Read the model definition and answer for the solid it produces. Units are mm, in the model's axes. A direction names the side the tool comes from. Round coordinates to 2 decimals unless told otherwise and drop trailing zeros. Loops run counter-clockwise (first coordinate to the right, second up) from the corner with the lowest first, then second, coordinate; pieces in that order, holes last. Notation, with made-up numbers: (39.5, 5) -> (64.5, 5) arc R25 cw to (64.5, 26) -> close; hole circle Ø11 at (-4.75, -11.75). An arc over 180 degrees is marked (long way). Put each result on its own line as item: value.
from build123d import *

# Parameters (mm, degrees)
F0_R     = 6.75
F1_DEPTH = 8
F3_DEPTH = 8.001


with BuildPart() as f1:
    # F0 (on Front) → F1 (new body)
    with BuildSketch(Plane.XZ):
        with Locations((-22.467263, 19.054513)):
            Circle(F0_R)
    extrude(amount=F1_DEPTH)

    # F2 (on face) → F3 (cut, through all)
    with BuildSketch(Plane.XZ.offset(8)):
        with BuildLine():
            Line((-22.467263, 20.554513), (-22.467263, 24.554513))
            ThreePointArc((-22.467263, 24.554513), (-24.660383, 24.098344), (-26.489708, 22.805504))
            Line((-26.489708, 22.805504), (-23.564294, 20.077511))
            ThreePointArc((-23.564294, 20.077511), (-23.065387, 20.430104), (-22.467263, 20.554513))
        make_face()
        with BuildLine():
            Line((-21.040678, 19.518039), (-17.236452, 20.754107))
            ThreePointArc((-17.236452, 20.754107), (-18.348007, 22.698924), (-20.142863, 24.039206))
            Line((-20.142863, 24.039206), (-21.833336, 20.413975))
            ThreePointArc((-21.833336, 20.413975), (-21.343829, 20.048443), (-21.040678, 19.518039))
        make_face()
        with BuildLine():
            ThreePointArc((-19.234444, 14.60492), (-17.728303, 16.263052), (-17.008259, 18.384232))
            Line((-17.008259, 18.384232), (-20.978444, 18.871709))
            ThreePointArc((-20.978444, 18.871709), (-21.174819, 18.293206), (-21.585585, 17.840988))
            Line((-21.585585, 17.840988), (-19.234444, 14.60492))
        make_face()
        with BuildLine():
            ThreePointArc((-25.700082, 14.60492), (-23.657681, 13.684885), (-21.417814, 13.655564))
            Line((-21.417814, 13.655564), (-22.18105, 17.582073))
            ThreePointArc((-22.18105, 17.582073), (-22.791922, 17.590069), (-23.348941, 17.840988))
            Line((-23.348941, 17.840988), (-25.700082, 14.60492))
        make_face()
        with BuildLine():
            Line((-23.893848, 19.518039), (-27.698074, 20.754107))
            ThreePointArc((-27.698074, 20.754107), (-27.941942, 18.527362), (-27.277671, 16.388061))
            Line((-27.277671, 16.388061), (-23.779193, 18.327299))
            ThreePointArc((-23.779193, 18.327299), (-23.960357, 18.910745), (-23.893848, 19.518039))
        make_face()
    extrude(amount=-F3_DEPTH, mode=Mode.SUBTRACT)


solid = f1.part
Item 1: Flat-ended cylindrical pins translate along their axes: pin 1 Ø3 at (y, z) = (-6.5, 14) entering from -X; pin 2 Ø6 at (x, z) = (-22.5, 23) entering from -Y; pin 3 Ø4.5 at (y, z) = (-6, 22.5) entering from -X; pin 4 Ø1 at (x, y) = (-24.5, -4.5) entering from +Z. Find the tip coordinate at first contact, or state that the pin passes through.
Derived:
pin 1: stops at x = -28.21
pin 2: stops at y = -8
pin 3: stops at x = -29.11
pin 4: stops at z = 25.63
Item 2: Which of the six approach directions +Z, -Z, +X, -X, +Y, -Y give full straight-line access (tool end or side, diameter ignored) to faces 3 (the flat face through (-25.553, -4.056, 17.344)), 4 (the flat face through (-23, 0, 19))?
Derived:
face 3: +Y, -Y
face 4: +Z, -Z, +X, -X, +Y
Item 3: Find the intervals of material crossed by line 1 along Z through (x, y) = (-22.5, -4.5); line 2 along Z through (x, y) = (-19.5, -4.25); line 3 along X through (y, z) = (-2.5, 23), in increasing order.
Derived:
line 1: z = 12.3 to 13.55, 17.55 to 20.55, 24.55 to 25.8
line 2: z = 12.99 to 14.97, 18.69 to 20.02, 23.69 to 25.12
line 3: x = -27.94 to -26.3, -22.47 to -20.63, -18.64 to -16.99
Item 4: For a pull along Z with two mould halves and no side action, classify faces 1 (the flat face through (-23, -8, 19)), 2 (the cylindrical face through (-17.74, -4.06, 16.24)) as pulls with the +Z half, pulls with the -Z half, needs draft (parallel to the pull), parting line crosses it, or undercut.
Derived:
face 1: needs draft
face 2: undercut
Item 5: The part is cut by section D-D (x = -27). Determine the outline of the cut face in (y, z), then the cut area to 3 significant figures.
Derived:
outline: (-8, 14.05) -> (0, 14.05) -> (0, 16.54) -> (-8, 16.54) -> close; (-8, 20.53) -> (0, 20.53) -> (0, 24.06) -> (-8, 24.06) -> close
area: 48.1 mm^2
Item 6: The part is cut by section B-B (z = 19.75). Determine the outline of the cut face in (x, y), then the cut area to 3 significant figures.
Derived:
outline: (-29.18, -8) -> (-27.92, -8) -> (-27.92, 0) -> (-29.18, 0) -> close; (-24.61, -8) -> (-21.14, -8) -> (-21.14, 0) -> (-24.61, 0) -> close; (-20.33, -8) -> (-15.75, -8) -> (-15.75, 0) -> (-20.33, 0) -> close
area: 74.4 mm^2
Item 7: The part is cut by section A-A (x = -19.5). Determine the outline of the cut face in (y, z), then the cut area to 3 significant figures.
Derived:
outline: (-8, 12.99) -> (0, 12.99) -> (0, 14.97) -> (-8, 14.97) -> close; (-8, 18.69) -> (0, 18.69) -> (0, 20.02) -> (-8, 20.02) -> close; (-8, 23.69) -> (0, 23.69) -> (0, 25.12) -> (-8, 25.12) -> close
area: 37.9 mm^2
Item 8: The part is cut by section C-C (y = -3.5). Determine the outline of the cut face in (x, z).
Derived:
outline: circle Ø13.5 at (-22.47, 19.05); hole (-27.7, 20.75) arc R5.5 ccw to (-27.28, 16.39) -> (-23.78, 18.33) arc R1.5 cw to (-23.89, 19.52) -> close; hole (-26.49, 22.81) -> (-23.56, 20.08) arc R1.5 cw to (-22.47, 20.55) -> (-22.47, 24.55) arc R5.5 ccw to start; hole (-25.7, 14.6) arc R5.5 ccw to (-21.42, 13.66) -> (-22.18, 17.58) arc R1.5 cw to (-23.35, 17.84) -> close; hole (-21.83, 20.41) arc R1.5 cw to (-21.04, 19.52) -> (-17.24, 20.75) arc R5.5 ccw to (-20.14, 24.04) -> close; hole (-21.59, 17.84) -> (-19.23, 14.6) arc R5.5 ccw to (-17.01, 18.38) -> (-20.98, 18.87) arc R1.5 cw to start
